Geometry check sheet. Reference: the model listing, model coordinates, mm. A direction names the side the tool comes from. Round coordinates to 2 decimals unless told otherwise and drop trailing zeros. Loops run counter-clockwise (first coordinate to the right, second up) from the corner with the lowest first, then second, coordinate; pieces in that order, holes last. Notation, with made-up numbers: (78, -2.5) -> (124, -2.5) arc R26 ccw to (124, 11.5) -> close; hole circle Ø10 at (-1, 42.5). An arc over 180 degrees is marked (long way). Use one line per item in the form item = value.
from build123d import *

# Parameters (mm, degrees)
BOSS_EXTRUDE1_DEPTH = 150
REVOLVE1_ANGLE      = 90
MIRROR1_ANGLE       = 90


# Read off the part's stored shape, not the designer's step: Mirror1
with BuildPart() as part:
    # Sketch2 → Boss-Extrude1 (new body)
    with BuildSketch(Plane(origin=(0, 0, 0), x_dir=(0, 0, -1), z_dir=(1, 0, 0))):
        with BuildLine():
            Line((0, 5), (0, -5))
            ThreePointArc((0, -5), (41.5, -46.5), (0, -88))
            Line((0, -88), (0, -92))
            ThreePointArc((0, -92), (43.037511543, -61.265588379), (27.932931003, -10.583410997))
            ThreePointArc((27.932931003, -10.583410997), (24.092356291, -2.052490679), (28.986658103, 5.920741122))
            ThreePointArc((28.986658103, 5.920741122), (54.98416934, 70.024683756), (0, 112))
            Line((0, 112), (0, 105))
            ThreePointArc((0, 105), (50, 55), (0, 5))
        make_face()
    extrude(amount=BOSS_EXTRUDE1_DEPTH)

    # Sketch2<2> → Revolve1 (revolve)
    with BuildSketch(Plane(origin=(0, 0, 0), x_dir=(0, 0, -1), z_dir=(1, 0, 0))):
        with BuildLine():
            Line((0, 5), (0, -5))
            ThreePointArc((0, -5), (41.5, -46.5), (0, -88))
            Line((0, -88), (0, -92))
            ThreePointArc((0, -92), (43.037511543, -61.265588379), (27.932931003, -10.583410997))
            ThreePointArc((27.932931003, -10.583410997), (24.092356291, -2.052490679), (28.986658103, 5.920741122))
            ThreePointArc((28.986658103, 5.920741122), (54.98416934, 70.024683756), (0, 112))
            Line((0, 112), (0, 105))
            ThreePointArc((0, 105), (50, 55), (0, 5))
        make_face()
    revolve(axis=Axis((0, 105, 0), (0, 1, 0)), revolution_arc=REVOLVE1_ANGLE)

    # Mirror1 outline → Mirror1 (revolve)
    with BuildSketch(Plane(origin=(150, 0, 0), x_dir=(1, 0, 0), z_dir=(0, 0, 1))):
        with BuildLine():
            ThreePointArc((28.986658103, 5.920741122), (54.98416934, 70.024683756), (0, 112))
            Line((0, 112), (0, 105))
            ThreePointArc((0, 105), (50, 55), (0, 5))
            Line((0, 5), (0, -5))
            ThreePointArc((0, -5), (41.5, -46.5), (0, -88))
            Line((0, -88), (0, -92))
            ThreePointArc((0, -92), (43.037511543, -61.265588379), (27.932931003, -10.583410997))
            ThreePointArc((27.932931003, -10.583410997), (24.092356291, -2.052490679), (28.986658103, 5.920741122))
        make_face()
    revolve(axis=Axis((150, 0, 0), (0, 1, 0)), revolution_arc=MIRROR1_ANGLE)


solid = part.part
1. Section check B-B (y = 55). Record the boundary of the cut face in (x, z).
Return value:
outline = (-57, 0) arc R57 ccw to (0, -57) -> (150, -57) arc R57 ccw to (207, 0) -> (200, 0) arc R50 cw to (150, -50) -> (0, -50) arc R50 cw to (-50, 0) -> close
2. Gauge pin test, flat ends, axial feed: pin 1 (1.5 mm diameter, centred on x = 164, y = -39.5, fed in from +Z); pin 2 (12 mm diameter, centred on x = -7, z = -11, fed in from -Y); pin 3 (10 mm diameter, centred on x = 89, y = -47.5, fed in from -Z). Record the tip position at first contact, or that the pin passes through.
Return value:
pin_1 = -38.12
pin_2 = -91.45
pin_3 = -45.5
3. Section check D-D (z = -53). Record the boundary of the cut face in (x, y), then the cut area to 3 significant figures.
Return value:
outline = (0, 34.02) -> (150, 34.02) arc R20.98 ccw to (150, 75.98) -> (0, 75.98) arc R20.98 ccw to start
area = 7,680 mm2
4. Tool access check on faces 1 (the cylindrical face through (73.95, -45.59, -41.49)), 2 (the cylindrical face through (73.95, -2.189, -24.085)). Record the directions out of +Z, -Z, +X, -X, +Y, -Y that give a thin tool (end or side, any length) a straight path to the whole face; none if there is none.
Return value:
face_1 = +Z
face_2 = -Z, +X, -X
5. Section check C-C (x = 38). Record the boundary of the cut face in (y, z), then the cut area to 3 significant figures.
Return value:
outline = (-92, 0) arc R45.5 ccw to (-10.58, -27.93) arc R10 cw to (5.92, -28.99) arc R57 ccw to (112, 0) -> (105, 0) arc R50 cw to (5, 0) -> (-5, 0) arc R41.5 cw to (-88, 0) -> close
area = 1,800 mm2
6. Section check A-A (z = -32). Record the boundary of the cut face in (x, y), then the cut area to 3 significant figures.
Return value:
outline = (0, -78.85) -> (150, -78.85) arc R32.35 ccw to (150, -14.15) -> (0, -14.15) arc R32.35 ccw to start; (0, 7.83) -> (150, 7.83) arc R47.17 ccw to (150, 102.17) -> (0, 102.17) arc R47.17 ccw to start; hole (0, -72.92) -> (150, -72.92) arc R26.42 ccw to (150, -20.08) -> (0, -20.08) arc R26.42 ccw to start; hole (0, 16.58) -> (150, 16.58) arc R38.42 ccw to (150, 93.42) -> (0, 93.42) arc R38.42 ccw to start
area = 7,850 mm2
7. Mould release check, pull along Y, two halves, no side actions. Record for faces 3 (the flat face through (74, 3, 0)), 4 (the cylindrical face through (73.95, 56.099, -49.988)): released by +Y, released by -Y, zero draft, split by the parting line, or undercut.
Return value:
face_3 = zero draft
face_4 = undercut
8. Material ranges on line 1 along Y through (x, z) = (153, -34); line 2 along Y through (x, z) = (-5, -38); line 3 along Y through (x, z) = (178, -31.5), recorded low to high.
Return value:
line_1 = -76.59 to -70.11, -22.89 to -16.41, 9.35 to 18.46, 91.54 to 100.65
line_2 = -71.02 to -62.41, -30.59 to -21.98, 12.81 to 22.89, 87.11 to 97.19
line_3 = -63.65 to -29.35, 16.62 to 28.1, 81.9 to 93.38
